from build123d import *


with BuildPart() as part:
    # Sketch2 → Revolve1 (revolve)
    with BuildSketch(Plane.XY):
        Polygon((-117, 0), (-98.142287974, 0), (-85, 10.210436502), (-85, 27.501263708), (-83, 27.501263708), (-83, 49.793455931), (-84.256609276, 49.793455931), (-84.256609276, 52.5), (-81.542630117, 52.5), (-81.542630117, 55.363879954), (-84.210889447, 55.363879954), (-84.210889447, 57.708994813), (-79.768205673, 60.5), (-75.979278114, 60.5), (-75.979278114, 53.479264493), (-74, 53.479264493), (-74, 48.88455903), (-79.768205673, 48.88455903), (-79.768205673, 33.88455903), (-74, 33.88455903), (-74, 26.204482528), (-75, 26.204482528), (-75, 12.93545297), (-69, 10.000926501), (-69, 6.929678014), (-75.818813089, 4.447833016), (-75.818813089, 2.344727047), (-70, 2.344727047), (-70, 1.144727047), (-71, 1.144727047), (-71, -24.879740451), (-77.75, -24.879740451), (-77.75, -17.379740451), (-74.5, -17.379740451), (-74.5, -2.65), (-80.647227673, -2.65), (-87.5, -9.277608288), (-87.5, -12), (-93.5, -12), (-93.5, -6), (-122, -6), (-122, -1.5), (-117, -1.5), align=None)
    revolve(axis=Axis((0, -27.768010488, 0), (0, 1, 0)))


solid = part.part
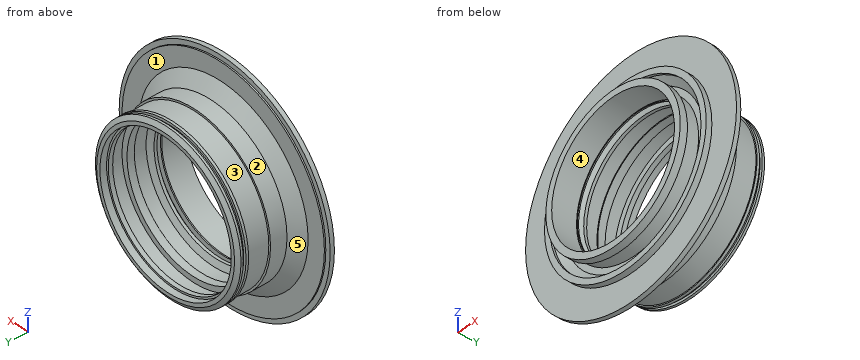
Input: part model. Units: mm. Frame: model coordinates. Face numbers are marked on the shaded views. A direction names the side the tool comes from. Give positions to 0.01 mm unless a question says otherwise; leave off trailing zeros. Order: outer loops, then holes, each group sorted by start corner. A loop starts at its lowest first (then second) coordinate and runs counter-clockwise, first axis right, second up. Notation, with made-up numbers: M 55,56 L 81,56 A21 ccw 81,77 Z; hole C 87,19.5 d1. An arc over 180 degrees is marked long. Answer as a JSON object with one key per item and string values.
1. Ray query, line 1 (Y direction, x = 22, z = 73); line 2 (X direction, y = -9, z = 62.5); line 3 (Z direction, x = 0, y = -9.9). Return the intervals inside material, ascending. Write a range as [from, to].
Result sheet:
{"line 1": "[-24.88, -17.38], [-2.65, 33.88], [48.88, 60.5]", "line 2": "[-69.54, -60.83], [-40.55, -33.69], [33.69, 40.55], [60.83, 69.54]", "line 3": "[-93.5, -87.5], [-74.5, -71], [71, 74.5], [87.5, 93.5]"}
2. Cut plane A-A, the plane y = 37. Output: boundary loops of the cut face in (x, z), and give its area (3 significant figures).
Result sheet:
{"outline": "C 0,0 d166; hole C 0,0 d159.54", "area": "1,650 mm²"}
3. Pull-direction query (Y, two-part tool) for the marked faces 1, 2 and 3; classes: +Y half, -Y half, draft (parallel to the pull), parting line (faces both ways), or undercut.
Result sheet:
{"face 1": "+Y half", "face 2": "draft", "face 3": "undercut"}
4. First-contact query: P1, Ø10, axis at x = -27.5, y = -4, coming from the -Z side; P2, Ø2, axis at y = 6, z = -39.5, coming from the +X side; P3, Ø4, axis at x = -57.5, z = 34.5, coming from the +Y side; P4, Ø4, axis at x = 11, z = -73.5, coming from the +Y side. Flat tips, straight axial feed; report the tip coordinate or a pass-through.
Result sheet:
{"P1": "z = -119.91", "P2": "x = 82.84", "P3": "y = 10.03", "P4": "y = 60.5"}
5. Reachability of the marked faces 4 and 5 from +Z, -Z, +X, -X, +Y, -Y: full face, straight path, thin tool, end or side. Return the list, or none.
Result sheet:
{"face 4": "-Y", "face 5": "+Y"}
6. Cut plane B-B, the plane z = 106. Output: boundary loops of the cut face in (x, y), and give its area (3 significant figures).
Result sheet:
{"outline": "M -60.4,-6 L 60.4,-6 L 60.4,-1.5 L 49.53,-1.5 L 49.53,0 L -49.53,0 L -49.53,-1.5 L -60.4,-1.5 Z", "area": "692 mm²"}
